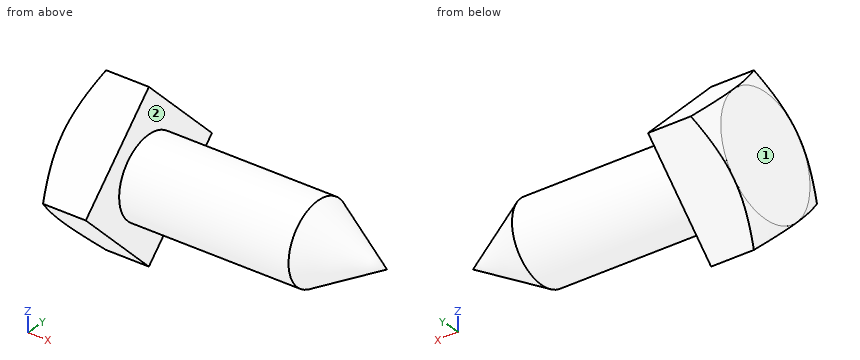
from build123d import *

# Parameters (mm, degrees)
SKETCH1_W      = 38.1
SKETCH1_H      = 38.1
BASEHEAD_DEPTH = 17.3736


with BuildPart() as part:
    # Sketch1 → BaseHead (new body)
    with BuildSketch(Plane(origin=(0, 0, 0), x_dir=(0, 0.7071067811865488, -0.7071067811865462), z_dir=(1, 0, 0))):
        Rectangle(SKETCH1_W, SKETCH1_H)
    extrude(amount=BASEHEAD_DEPTH)

    # Sketch2 → Body (revolve)
    with BuildSketch(Plane.XY, mode=Mode.PRIVATE) as body_sk:
        Polygon((17.3736, 0), (17.3736, 12.7), (71.576554744, 12.7), (93.5736, 0), align=None)
    revolve(body_sk.sketch.rotate(Axis((0, 0, 0), (1, 0, 0)), 90), axis=Axis((0, 0, 0), (1, 0, 0)))

    # Sketch3 → HeadChamfer (revolve, cut)
    with BuildSketch(Plane.XY):
        Polygon((0, 19.05), (-12.7, 19.05), (-12.7, 52.340768363), (15.523740234, 52.340768363), align=None)
    revolve(axis=Axis((0, 0, 0), (1, 0, 0)), mode=Mode.SUBTRACT)


solid = part.part
Work out the finished part from the listing and answer in its coordinate system (mm). Face numbers are marked on the shaded views. A direction names the side the tool comes from. Give positions to 0.01 mm unless a question says otherwise; leave off trailing zeros. Order: outer loops, then holes, each group sorted by start corner. A loop starts at its lowest first (then second) coordinate and runs counter-clockwise, first axis right, second up. Notation, with made-up numbers: M 71.5,26.25 L 105.5,26.25 A12 cw 105.5,30.25 Z; hole C 42.25,60 d1. An arc over 180 degrees is marked long. Return JSON: item names as keys, results as strings.
Q1. Each of these flat-tipped pins is pushed along its axis until it touches: pin 1 (5 mm diameter, centred on x = 47, z = 8.5, fed in from -Y); pin 2 (5 mm diameter, centred on x = 26.5, y = -4, fed in from +Z); pin 3 (5 mm diameter, centred on x = 12.5, y = 4, fed in from +Z). Where does it stop, or does it pass through?
Answer below:
{"pin 1": "stops at y = -11.19", "pin 2": "stops at z = 12.61", "pin 3": "stops at z = 25.44"}
Q2. Find section A-A, the plane x = 9. Write down the section's boundary in (y, z).
Answer below:
{"outline": "M -26.94,0 L 0,-26.94 L 26.94,0 L 0,26.94 Z"}
Q3. Find section C-C, the plane x = 84. Write down the section's boundary in (y, z), and give its area (3 significant figures).
Answer below:
{"outline": "C 0,0 d11.05", "area": "96.0 mm^2"}
Q4. Find section B-B, the plane x = 29.5. Write down the section's boundary in (y, z).
Answer below:
{"outline": "C 0,0 d25.4"}
Q5. Find the intervals of material crossed by line 1 along X through (y, z) = (-16.5, -8.5); line 2 along Y through (x, z) = (8.5, -8); line 3 along X through (y, z) = (-4, 8), in increasing order. Write a range as [from, to].
Answer below:
{"line 1": "x = [0, 17.37]", "line 2": "y = [-18.94, 18.94]", "line 3": "x = [0, 78.08]"}
Q6. Which of the six approach directions +Z, -Z, +X, -X, +Y, -Y give full straight-line access (tool end or side, diameter ignored) to the marked faces 1 and 2?
Answer below:
{"face 1": "+Z, -Z, -X, +Y, -Y", "face 2": "+X"}
